from build123d import *

# Parameters (mm, degrees)
SKETCH1_R           = 9.4615
SKETCH1_R_2         = 1.778
BOSS_EXTRUDE1_DEPTH = 3.175
SKETCH2_R           = 10.7315
SKETCH2_R_2         = 9.4615
BOSS_EXTRUDE2_DEPTH = 1.905
CHAMFER1_SIZE       = 0.254
SKETCH3_R           = 9.4615
SKETCH3_R_2         = 8.8265
BOSS_EXTRUDE3_DEPTH = 4.7625
CHAMFER2_SIZE       = 0.254
SKETCH4_R           = 8.8265
SKETCH4_R_2         = 6.985
BOSS_EXTRUDE4_DEPTH = 4.2545
SKETCH5_R           = 6.985
SKETCH5_R_2         = 6.35
BOSS_EXTRUDE5_DEPTH = 4.7625
CHAMFER3_SIZE       = 0.254


with BuildPart() as part:
    # Sketch1 → Boss-Extrude1 (new body)
    with BuildSketch(Plane(origin=(0, 0, 0), x_dir=(1, 0, 0), z_dir=(0, 1, 0))):
        with BuildLine():
            Line((-15.113, -16.6497), (-15.113, -15.742069175))
            Line((-15.113, -15.742069175), (-8.537191562, -10.640953872))
            ThreePointArc((-8.537191562, -10.640953872), (-7.177584853, -10.115559905), (-5.753021125, -10.424084468))
            ThreePointArc((-5.753021125, -10.424084468), (0, -11.90625), (5.753021125, -10.424084468))
            ThreePointArc((5.753021125, -10.424084468), (7.177584853, -10.115559905), (8.537191562, -10.640953872))
            Line((8.537191562, -10.640953872), (15.113, -15.742069175))
            Line((15.113, -15.742069175), (15.113, -16.6497))
            Line((15.113, -16.6497), (21.463, -16.6497))
            Line((21.463, -16.6497), (21.463, -10.2997))
            Line((21.463, -10.2997), (18.457244016, -10.2997))
            Line((18.457244016, -10.2997), (12.429339722, -5.623615663))
            ThreePointArc((12.429339722, -5.623615663), (11.582420607, -4.43732007), (11.527087077, -2.980780533))
            ThreePointArc((11.527087077, -2.980780533), (11.90625, 0), (11.527087077, 2.980780533))
            ThreePointArc((11.527087077, 2.980780533), (11.582420607, 4.43732007), (12.429339722, 5.623615663))
            Line((12.429339722, 5.623615663), (18.457244016, 10.2997))
            Line((18.457244016, 10.2997), (21.463, 10.2997))
            Line((21.463, 10.2997), (21.463, 16.6497))
            Line((21.463, 16.6497), (15.113, 16.6497))
            Line((15.113, 16.6497), (15.113, 15.742069175))
            Line((15.113, 15.742069175), (8.537191562, 10.640953872))
            ThreePointArc((8.537191562, 10.640953872), (7.177584853, 10.115559905), (5.753021125, 10.424084468))
            ThreePointArc((5.753021125, 10.424084468), (0, 11.90625), (-5.753021125, 10.424084468))
            ThreePointArc((-5.753021125, 10.424084468), (-7.177584853, 10.115559905), (-8.537191562, 10.640953872))
            Line((-8.537191562, 10.640953872), (-15.113, 15.742069175))
            Line((-15.113, 15.742069175), (-15.113, 16.6497))
            Line((-15.113, 16.6497), (-21.463, 16.6497))
            Line((-21.463, 16.6497), (-21.463, 10.2997))
            Line((-21.463, 10.2997), (-18.457244016, 10.2997))
            Line((-18.457244016, 10.2997), (-12.429339722, 5.623615663))
            ThreePointArc((-12.429339722, 5.623615663), (-11.582420607, 4.43732007), (-11.527087077, 2.980780533))
            ThreePointArc((-11.527087077, 2.980780533), (-11.90625, 0), (-11.527087077, -2.980780533))
            ThreePointArc((-11.527087077, -2.980780533), (-11.582420607, -4.43732007), (-12.429339722, -5.623615663))
            Line((-12.429339722, -5.623615663), (-18.457244016, -10.2997))
            Line((-18.457244016, -10.2997), (-21.463, -10.2997))
            Line((-21.463, -10.2997), (-21.463, -16.6497))
            Line((-21.463, -16.6497), (-15.113, -16.6497))
        make_face()
        with Locations(Location((0, 0, 0), (0, 0, 270))):
            Circle(SKETCH1_R, mode=Mode.SUBTRACT)
        with Locations(Location((-18.288, -13.4747, 0), (0, 0, 270))):
            Circle(SKETCH1_R_2, mode=Mode.SUBTRACT)
        with Locations(Location((-18.288, 13.4747, 0), (0, 0, 270))):
            Circle(SKETCH1_R_2, mode=Mode.SUBTRACT)
        with Locations(Location((18.288, -13.4747, 0), (0, 0, 270))):
            Circle(SKETCH1_R_2, mode=Mode.SUBTRACT)
        with Locations(Location((18.288, 13.4747, 0), (0, 0, 270))):
            Circle(SKETCH1_R_2, mode=Mode.SUBTRACT)
    extrude(amount=BOSS_EXTRUDE1_DEPTH)

    # Sketch2 → Boss-Extrude2 (add)
    with BuildSketch(Plane(origin=(0, 3.175, 0), x_dir=(1, 0, 0), z_dir=(0, 1, 0))):
        with Locations(Location((0, 0, 0), (0, 0, 90))):
            Circle(SKETCH2_R)
        with Locations(Location((0, 0, 0), (0, 0, 270))):
            Circle(SKETCH2_R_2, mode=Mode.SUBTRACT)
    extrude(amount=BOSS_EXTRUDE2_DEPTH)

    # Chamfer1
    chamfer1_edges = [part.edges().sort_by_distance(p)[0] for p in [
        (0, 5.08, -9.4615),
        (0, 0, -9.4615),
    ]]
    chamfer(chamfer1_edges, length=CHAMFER1_SIZE)



with BuildPart() as body_2:
    # Sketch3 → Boss-Extrude3 (new body)
    with BuildSketch(Plane(origin=(0, 5.08, 0), x_dir=(1, 0, 0), z_dir=(0, 1, 0))):
        with Locations(Location((0, 0, 0), (0, 0, 270))):
            Circle(SKETCH3_R)
        with Locations(Location((0, 0, 0), (0, 0, 270))):
            Circle(SKETCH3_R_2, mode=Mode.SUBTRACT)
    extrude(amount=-BOSS_EXTRUDE3_DEPTH)

    # Chamfer2
    chamfer2_edges = [body_2.edges().sort_by_distance(p)[0] for p in [
        (0, 0.3175, -8.8265),
        (0, 5.08, -8.8265),
    ]]
    chamfer(chamfer2_edges, length=CHAMFER2_SIZE)


with BuildPart() as part_1:
    add(part.part)

    add(body_2.part)  # Boss-Extrude4 merges body 2
    # Sketch4 → Boss-Extrude4 (add)
    with BuildSketch(Plane(origin=(0, 4.826, 0), x_dir=(-1, 0, 0), z_dir=(0, 1, 0))):
        Circle(SKETCH4_R)
        with Locations(Location((0, 0, 0), (0, 0, 90))):
            Circle(SKETCH4_R_2, mode=Mode.SUBTRACT)
    extrude(amount=-BOSS_EXTRUDE4_DEPTH)

    # Sketch5 → Boss-Extrude5 (add)
    with BuildSketch(Plane(origin=(0, 5.08, 0), x_dir=(1, 0, 0), z_dir=(0, 1, 0))):
        with Locations(Location((0, 0, 0), (0, 0, 270))):
            Circle(SKETCH5_R)
        with Locations(Location((0, 0, 0), (0, 0, 270))):
            Circle(SKETCH5_R_2, mode=Mode.SUBTRACT)
    extrude(amount=-BOSS_EXTRUDE5_DEPTH)

    # Chamfer3
    chamfer3_edges = [part_1.edges().sort_by_distance(p)[0] for p in [
        (0, 0.3175, -6.985),
        (0, 5.08, -6.985),
    ]]
    chamfer(chamfer3_edges, length=CHAMFER3_SIZE - 0.0001)  # a hair under: the kernel refuses the full size


solid = part_1.part
Read the model definition and answer for the solid it produces. Units are mm, in the model's axes. A direction names the side the tool comes from. Coordinates: 2 decimals unless noted, no trailing zeros. Order: outer loops, then holes, each group sorted by start corner. A loop starts at its lowest first (then second) coordinate and runs counter-clockwise, first axis right, second up. Notation, with made-up numbers: M 17,79.25 L 47,79.25 A31 ccw 47,103.25 Z; hole C -26.75,-19 d1. An arc over 180 degrees is marked long. Put each result on its own line as item: value. Start each with the question number.
Item 1: The mould has two halves that part along Z. Classify faces 4 (the face through (-10, 5.08, 2)), 5 (the face through (0.084, 1.565, -11.906)), 6 (the face through (-20, 2, 10.3)): +Z half, -Z half, draft (parallel to the pull), parting line (faces both ways), or undercut.
Item 2: Section C-C, the plane y = 4.15 is taken. Determine the outline of the cut face in (x, z).
Item 3: For faces 1 (the face through (20, 2, -10.3)), 2 (the face through (-15.113, 2, -16)), 3 (the face through (7.8, 0.317, -5)), determine the directions among +Z, -Z, +X, -X, +Y, -Y from which every point of the face is accessible in a straight line to the end or side of a thin tool.
Item 4: Consider probe 1 along X at (y, z) = (3.75, 0); probe 2 along X at (y, z) = (2.3, 11); probe 3 along Z at (x, y) = (-17, 2.8). Determine where each line is inside the solid, lowest interval first. Write a range as [from, to].
Item 5: Section A-A, the plane z = 14.5 is taken. Determine the outline of the cut face in (x, y) (3 decimals).
Item 6: Section B-B, the plane x = -14 is taken. Determine the outline of the cut face in (y, z) (3 decimals), plus the area to 3 significant figures.
Item 7: Given pin 1 Ø10 at (x, z) = (4, -6.5) entering from +Y; pin 2 Ø1 at (x, y) = (-9, 1) entering from +Z; pin 3 Ø4.5 at (x, z) = (18.29, 13.47) entering from +Y (3 decimals); pin 4 Ø2 at (x, y) = (-10.5, 3) entering from +Z, each flat-ended and moving along its own axis, determine where each tip first touches the part or whether it passes through.
Computed:
1. face 4: draft
1. face 5: -Z half
1. face 6: undercut
2. outline: C 0,0 d21.46; hole C 0,0 d12.7
3. face 1: +X, +Y, -Y
3. face 2: -Z, +Y, -Y
3. face 3: -Y
4. probe 1: x = [-10.73, -6.35], [6.35, 10.73]
4. probe 2: x = [-21.46, -9], [-4.56, 4.56], [9, 21.46]
4. probe 3: z = [-16.65, -14.7], [-12.25, -9.17], [9.17, 12.25], [14.7, 16.65]
5. outline: M -21.463,0 L -19.741,0 L -19.741,3.175 L -21.463,3.175 Z; M -16.835,0 L -13.512,0 L -13.512,3.175 L -16.835,3.175 Z; M 13.512,0 L 16.835,0 L 16.835,3.175 L 13.512,3.175 Z; M 19.741,0 L 21.463,0 L 21.463,3.175 L 19.741,3.175 Z
6. outline: M 0,-14.879 L 3.175,-14.879 L 3.175,-6.842 L 0,-6.842 Z; M 0,6.842 L 3.175,6.842 L 3.175,14.879 L 0,14.879 Z
6. area: 51.0 mm2
7. pin 1: stops at y = 5.08
7. pin 2: stops at z = 11.39
7. pin 3: stops at y = 3.175
7. pin 4: stops at z = 12.94
